Job drawing, mm, ordinate dimensions from the low corner. One solid piece. Round coordinates to 2 decimals unless told otherwise and drop trailing zeros. Loops run counter-clockwise (first coordinate to the right, second up) from the corner with the lowest first, then second, coordinate; pieces in that order, holes last. Notation, with made-up numbers: M 75,-9 L 121,-9 A13 cw 121,12 Z; hole C 50,12 d4. An arc over 180 degrees is marked long. Use one line per item in the form item = value.
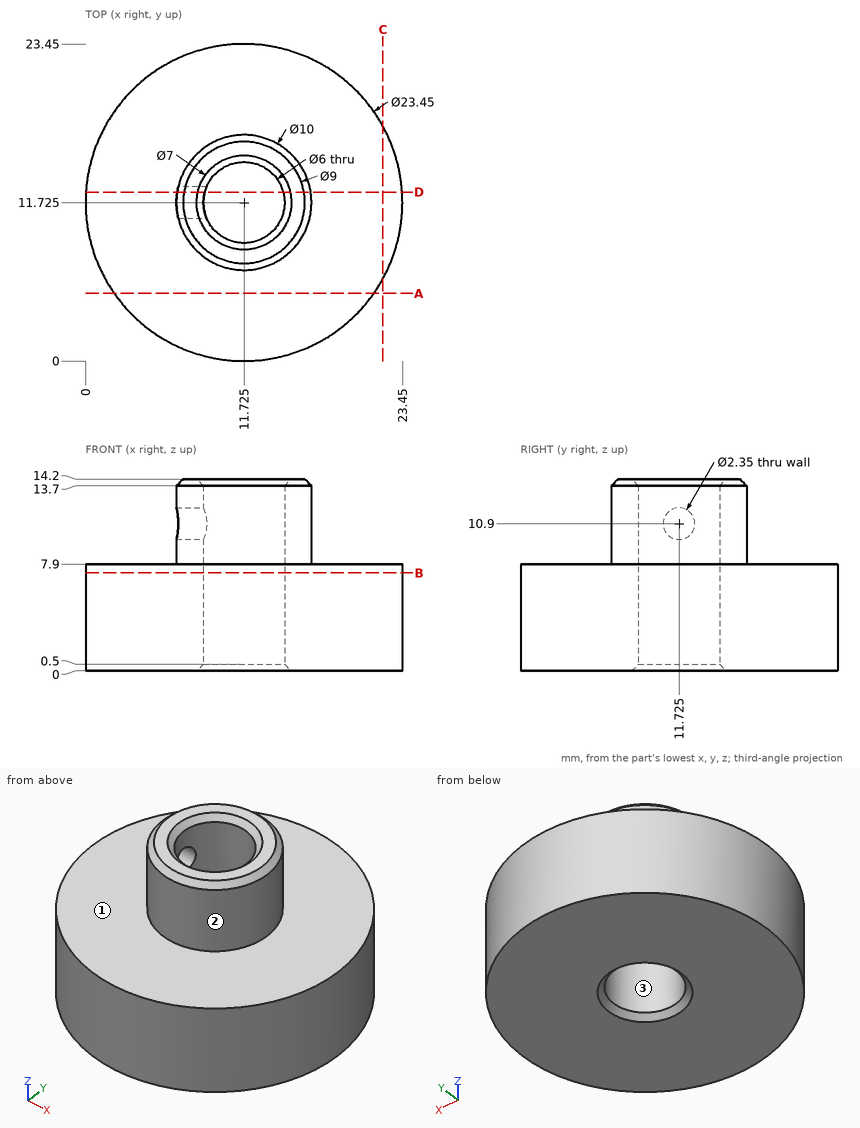
1. Drop flat-ended pins along their axis: P1, Ø7, axis at x = 6, y = 12.5, coming from the +Z side; P2, Ø3, axis at y = 16, z = 2, coming from the +X side; P3, Ø3, axis at x = 4, z = 5, coming from the -Y side; P4, Ø2, axis at y = 11.725, z = 10.9, coming from the -X side. Give the stop position or say it passes through.
Completed:
P1 = 14.2
P2 = 23.12
P3 = 1.79
P4 = 14.55
2. Cut at B-B on z = 7.25. Write the cut outline in (x, y) (3 decimals), and give its area (3 significant figures).
Completed:
outline = C 11.725,11.725 d23.45; hole C 11.725,11.725 d6
area = 404 mm2
3. Probe line 1 along Z through (x, y) = (7.5, 20.5); line 2 along X through (y, z) = (12.75, 12.75); line 3 along X through (y, z) = (8.25, 9.5). List the from-to ranges inside material, lowest first. Write a range as from..to.
Completed:
line_1 = 0..7.9
line_2 = 6.83..8.91, 14.54..16.62
line_3 = 8.13..15.32
4. Cut at A-A on y = 5. Write the cut outline in (x, z).
Completed:
outline = M 2.12,0 L 21.33,0 L 21.33,7.9 L 2.12,7.9 Z
5. Cut at D-D on y = 12.5. State how many separate pieces and enclosed holes the cut face has, and give its area (3 significant figures).
Completed:
separate_pieces = 3
enclosed_holes = 0
area = 160 mm2
6. Cut at C-C on x = 22. Write the cut outline in (y, z), and give its area (3 significant figures).
Completed:
outline = M 6.08,0 L 17.37,0 L 17.37,7.9 L 6.08,7.9 Z
area = 89.2 mm2
7. Pull direction Y, two halves, no side cores. Call the marked faces 1, 2 and 3: +Y half, -Y half, draft (parallel to the pull), parting line (faces both ways), or undercut.
Completed:
face_1 = draft
face_2 = parting line
face_3 = undercut
